```python
from build123d import *

# Parameters (mm, degrees)
BOSS_EXTRUDE1_DEPTH  = 2
M2_CLEARANCE_HOLE1_D = 2.6
BOSS_EXTRUDE2_START  = 7.6
BOSS_EXTRUDE2_DEPTH  = 7.6
SKETCH9_W            = 24
SKETCH9_H            = 2.4
CUT_EXTRUDE1_DEPTH   = 2


with BuildPart() as part:
    # Sketch1 → Boss-Extrude1 (new body)
    with BuildSketch(Plane(origin=(0, 0, 0), x_dir=(1, 0, 0), z_dir=(0, 1, 0))):
        with BuildLine():
            Line((-63.5, 0), (-53.5, 0))
            Line((-53.5, 0), (53.5, 0))
            Line((53.5, 0), (63.5, 0))
            Line((63.5, 0), (63.5, 17.78))
            ThreePointArc((63.5, 17.78), (59.780256121, 26.760256121), (50.8, 30.48))
            Line((50.8, 30.48), (-50.8, 30.48))
            ThreePointArc((-50.8, 30.48), (-59.780256121, 26.760256121), (-63.5, 17.78))
            Line((-63.5, 17.78), (-63.5, 0))
        make_face()
        with BuildLine():
            Line((-53.5, 2.4), (-53.5, 20.08))
            ThreePointArc((-53.5, 20.08), (-51.156854249, 25.736854249), (-45.5, 28.08))
            Line((-45.5, 28.08), (45.5, 28.08))
            ThreePointArc((45.5, 28.08), (51.156854249, 25.736854249), (53.5, 20.08))
            Line((53.5, 20.08), (53.5, 2.4))
            Line((53.5, 2.4), (-53.5, 2.4))
        make_face(mode=Mode.SUBTRACT)
    extrude(amount=BOSS_EXTRUDE1_DEPTH)

    # M2 Clearance Hole1 (through all)
    with Locations(Plane(origin=(0, 2, 0), x_dir=(1, 0, 0), z_dir=(0, 1, 0))):
        with Locations((-58.42, 11.43), (58.42, 11.43)):
            Hole(M2_CLEARANCE_HOLE1_D / 2)

    # Sketch8 → Boss-Extrude2 (add)
    with BuildSketch(Plane(origin=(0, 0, 0), x_dir=(-1, 0, 0), z_dir=(0, -1, 0)).offset(BOSS_EXTRUDE2_START)):
        with BuildLine():
            Line((63.5, 0), (63.5, 17.78))
            ThreePointArc((63.5, 17.78), (59.780256121, 26.760256121), (50.8, 30.48))
            Line((50.8, 30.48), (-50.8, 30.48))
            ThreePointArc((-50.8, 30.48), (-59.780256121, 26.760256121), (-63.5, 17.78))
            Line((-63.5, 17.78), (-63.5, 0))
            Line((-63.5, 0), (63.5, 0))
        make_face()
        with BuildLine():
            Line((-61.1, 2.4), (61.1, 2.4))
            Line((61.1, 2.4), (61.1, 17.78))
            ThreePointArc((61.1, 17.78), (58.083199846, 25.063199846), (50.8, 28.08))
            Line((50.8, 28.08), (-50.8, 28.08))
            ThreePointArc((-50.8, 28.08), (-58.083199846, 25.063199846), (-61.1, 17.78))
            Line((-61.1, 17.78), (-61.1, 2.4))
        make_face(mode=Mode.SUBTRACT)
    extrude(amount=-BOSS_EXTRUDE2_DEPTH)

    # Sketch9 → Cut-Extrude1 (cut)
    with BuildSketch(Plane(origin=(0, 2, 0), x_dir=(1, 0, 0), z_dir=(0, 1, 0))):
        with Locations((0, 1.2)):
            Rectangle(SKETCH9_W, SKETCH9_H)
    extrude(amount=-CUT_EXTRUDE1_DEPTH, mode=Mode.SUBTRACT)


solid = part.part
```
Geometry check sheet. Reference: the model listing, model coordinates, mm. A direction names the side the tool comes from. Coordinates: 2 decimals unless noted, no trailing zeros. Order: outer loops, then holes, each group sorted by start corner. A loop starts at its lowest first (then second) coordinate and runs counter-clockwise, first axis right, second up.
Q1. Sectioned sample at A-A on x = 32. Record the cut outline in (y, z).
Reply:
outline: (-7.6, -30.48) - (2, -30.48) - (2, -28.08) - (-7.6, -28.08) - close; (-7.6, -2.4) - (2, -2.4) - (2, 0) - (-7.6, 0) - close
Q2. Tool access check on faces 1 (the face through (-12, 1, -1)), 2 (the face through (4, 2, -29)), 3 (the face through (-57, 0, -15)), 4 (the face through (51.094, 0.986, -25.799)). Record the directions out of +Z, -Z, +X, -X, +Y, -Y that give a thin tool (end or side, any length) a straight path to the whole face; none if there is none.
Reply:
face 1: +Z, +Y
face 2: +Z, -Z, +X, -X, +Y
face 3: -Y
face 4: +Y, -Y
Q3. Sectioned sample at D-D on z = -24. Record the cut outline in (x, y).
Reply:
outline: (-61.87, -7.6) - (-59.01, -7.6) - (-59.01, 0) - (-52.47, 0) - (-52.47, 2) - (-61.87, 2) - close; (52.47, 0) - (59.01, 0) - (59.01, -7.6) - (61.87, -7.6) - (61.87, 2) - (52.47, 2) - close
Q4. Depth check by flat-ended pin: pin 1 Ø12 at (x, z) = (36.5, -24.5) entering from -Y; pin 2 Ø2.5 at (x, z) = (6, -1) entering from +Y; pin 3 Ø12.5 at (x, z) = (54.5, -13.5) entering from -Y. Enter the tip coordinate at first touch or a pass-through.
Reply:
pin 1: stops at y = -7.6
pin 2: stops at y = 0
pin 3: stops at y = 0
Q5. Sectioned sample at B-B on z = -11.43. Record the cut outline in (x, y).
Reply:
outline: (-63.5, -7.6) - (-61.1, -7.6) - (-61.1, 0) - (-59.72, 0) - (-59.72, 2) - (-63.5, 2) - close; (-57.12, 0) - (-53.5, 0) - (-53.5, 2) - (-57.12, 2) - close; (53.5, 0) - (57.12, 0) - (57.12, 2) - (53.5, 2) - close; (59.72, 0) - (61.1, 0) - (61.1, -7.6) - (63.5, -7.6) - (63.5, 2) - (59.72, 2) - close
Q6. Thickness scan on probe 1 along X at (y, z) = (1.1, -11.43); probe 2 along Z at (x, y) = (-4.5, -2.5); probe 3 along X at (y, z) = (-4.5, -2.5). Record the ranges inside material, lowest first.
Reply:
probe 1: x = -63.5 to -59.72, -57.12 to -53.5, 53.5 to 57.12, 59.72 to 63.5
probe 2: z = -30.48 to -28.08, -2.4 to 0
probe 3: x = -63.5 to -61.1, 61.1 to 63.5
Q7. Draft check along X on faces 5 (the face through (58.003, -3.853, -25.143)), 6 (the face through (-1, -3, -30.48)), 7 (the face through (-59.88, -2.87, -26.66)). Enter one of: released by +X, released by -X, zero draft, split by the parting line, or undercut.
Reply:
face 5: undercut
face 6: zero draft
face 7: released by -X
Q8. Sectioned sample at C-C on y = -2. Record the cut outline in (x, z).
Reply:
outline: (-63.5, -17.78) arc R12.7 ccw to (-50.8, -30.48) - (50.8, -30.48) arc R12.7 ccw to (63.5, -17.78) - (63.5, 0) - (-63.5, 0) - close; hole (-61.1, -17.78) arc R10.3 ccw to (-50.8, -28.08) - (50.8, -28.08) arc R10.3 ccw to (61.1, -17.78) - (61.1, -2.4) - (-61.1, -2.4) - close
